from build123d import *

# Parameters (mm, degrees)
BOSS_EXTRUDE1_DEPTH = 4


with BuildPart() as part:
    # Sketch1 → Boss-Extrude1 (new body)
    with BuildSketch(Plane.XY):
        with BuildLine():
            Line((-120, -99), (-120, 99))
            Line((-120, 99), (120, 99))
            Line((120, 99), (120, -99))
            Line((120, -99), (100, -99))
            Line((100, -99), (83.00243962, -77.753049524))
            ThreePointArc((83.00243962, -77.753049524), (79.52563883, -74.986967637), (75.193751525, -74))
            Line((75.193751525, -74), (-75.193751525, -74))
            ThreePointArc((-75.193751525, -74), (-79.52563883, -74.986967637), (-83.00243962, -77.753049524))
            Line((-83.00243962, -77.753049524), (-100, -99))
            Line((-100, -99), (-120, -99))
        make_face()
    extrude(amount=BOSS_EXTRUDE1_DEPTH)


solid = part.part
Work out the finished part from the listing and answer in its coordinate system (mm). A direction names the side the tool comes from. Coordinates: 2 decimals unless noted, no trailing zeros. Order: outer loops, then holes, each group sorted by start corner. A loop starts at its lowest first (then second) coordinate and runs counter-clockwise, first axis right, second up. Notation, with made-up numbers: (12.25, 47) - (71.25, 47) arc R31 ccw to (71.25, 74) - close; hole circle Ø10 at (56.25, 35). An arc over 180 degrees is marked (long way). Put each result on its own line as item: value. Start each with the question number.
1) Find section B-B (z = 3.05). Give the vertices of the cut face in (x, y).
2) For a pull along X with two mould halves and no side action, classify faces 1 (the flat face through (2, 1, 0)), 2 (the flat face through (92, -89, 2)) as released by +X, released by -X, zero draft, split by the parting line, or undercut.
3) For faces 3 (the flat face through (-91.382, -88.228, 1.972)), 4 (the flat face through (2, 1, 4)), determine the directions among +Z, -Z, +X, -X, +Y, -Y from which every point of the face is accessible in a straight line to the end or side of a thin tool.
4) Find section C-C (x = -89). Give the vertices of the cut face in (y, z), plus the area to 3 significant figures.
5) Flat-ended cylindrical pins translate along their axes: pin 1 (6 mm diameter, centred on x = -14.5, y = -8.5, fed in from -Z); pin 2 (2 mm diameter, centred on x = 19, z = 3, fed in from -Y). Find the tip coordinate at first contact, or state that the pin passes through.
6) Find section A-A (y = -82.5). Give the vertices of the cut face in (x, z).
7) Find the intervals of material crossed by line 1 (Y direction, x = -62, z = 0.8); line 2 (Y direction, x = 95, z = 2.9), in increasing order. Write a range as from..to.
8) Find section D-D (x = 5). Give the vertices of the cut face in (y, z), plus the area to 3 significant figures.
Results list:
1. outline: (-120, -99) - (-100, -99) - (-83, -77.75) arc R10 cw to (-75.19, -74) - (75.19, -74) arc R10 cw to (83, -77.75) - (100, -99) - (120, -99) - (120, 99) - (-120, 99) - close
2. face 1: zero draft
2. face 2: undercut
3. face 3: +Z, -Z, -Y
3. face 4: +Z, +X, -X, +Y, -Y
4. outline: (-85.25, 0) - (99, 0) - (99, 4) - (-85.25, 4) - close
4. area: 737 mm^2
5. pin 1: stops at z = 0
5. pin 2: stops at y = -74
6. outline: (-120, 0) - (-86.8, 0) - (-86.8, 4) - (-120, 4) - close; (86.8, 0) - (120, 0) - (120, 4) - (86.8, 4) - close
7. line 1: y = -74..99
7. line 2: y = -92.75..99
8. outline: (-74, 0) - (99, 0) - (99, 4) - (-74, 4) - close
8. area: 692 mm^2
